from build123d import *

# Parameters (mm, degrees)
SKETCH1_R                                           = 50.375
BOSS_EXTRUDE1_DEPTH                                 = 7
SKETCH3_R                                           = 18.5
CUT_EXTRUDE2_DEPTH                                  = 72.584085173
CBORE_FOR_M3_HEX_SOCKET_HEAD_CAP_SCREW1_D           = 3.4
CBORE_FOR_M3_HEX_SOCKET_HEAD_CAP_SCREW1_CBORE_D     = 6.5
CBORE_FOR_M3_HEX_SOCKET_HEAD_CAP_SCREW1_CBORE_DEPTH = 3.4
CIRPATTERN1_COUNT                                   = 15


with BuildPart() as part:
    # Sketch1 → Boss-Extrude1 (new body)
    with BuildSketch(Plane.XY):
        Circle(SKETCH1_R)
    extrude(amount=BOSS_EXTRUDE1_DEPTH)

    # Sketch3 → Cut-Extrude2 (cut, through all)
    with BuildSketch(Plane.XY.offset(7)):
        Circle(SKETCH3_R)
    extrude(amount=-CUT_EXTRUDE2_DEPTH, mode=Mode.SUBTRACT)

    # CBORE for M3 Hex Socket Head Cap Screw1 (through all)
    with Locations(Plane.XY.offset(7)):
        with Locations((0, 40)):
            cbore_for_m3_hex_socket_head_cap_screw1 = CounterBoreHole(CBORE_FOR_M3_HEX_SOCKET_HEAD_CAP_SCREW1_D / 2, CBORE_FOR_M3_HEX_SOCKET_HEAD_CAP_SCREW1_CBORE_D / 2, CBORE_FOR_M3_HEX_SOCKET_HEAD_CAP_SCREW1_CBORE_DEPTH)

    # CirPattern1: CBORE for M3 Hex Socket Head Cap Screw1 ×15 about axis
    cirpattern1_axis = Axis((0, 0, 0), (0, 0, 1))
    for i in range(1, CIRPATTERN1_COUNT):
        add(cbore_for_m3_hex_socket_head_cap_screw1.rotate(cirpattern1_axis, i * 360 / CIRPATTERN1_COUNT), mode=Mode.SUBTRACT)


solid = part.part
For this review, take the finished solid that the model builds, in its own axes (mm). A direction names the side the tool comes from. Give positions to 0.01 mm unless a question says otherwise; leave off trailing zeros. Order: outer loops, then holes, each group sorted by start corner. A loop starts at its lowest first (then second) coordinate and runs counter-clockwise, first axis right, second up. Notation, with made-up numbers: (-36, 13) - (-19, 13) arc R17 ccw to (-19, 37) - close; hole circle Ø2 at (55.25, 57.25). An arc over 180 degrees is marked (long way). Answer as a JSON object with one key per item and string values. Group by question number.
Item 1: Wall thickness on line 1 along Y through (x, z) = (0, 1.2) (3 decimals); line 2 along X through (y, z) = (9.5, 6.5); line 3 along X through (y, z) = (25.5, 4): over which ranges is each line inside the solid? List them lowest first.
Item 2: Clearance check with flat-ended pins moving along their axes: pin 1 Ø5.5 at (x, y) = (-23.51, -32.36) entering from -Z; pin 2 Ø4 at (x, y) = (0, 40) entering from +Z; pin 3 Ø1.5 at (y, z) = (-33.5, 5.5) entering from -X; pin 4 Ø3 at (x, z) = (-30.5, 2.5) entering from +Y. State where each tip first meets the part, or that it passes through.
Item 3: Take a section at B-B on y = -20. Give the boundary of the cut face in (x, z).
Item 4: Take a section at A-A on x = 0. Give the boundary of the cut face in (y, z) (3 decimals), and give its area (3 significant figures).
Item 5: Machinability: for faces 1 (the cylindrical face through (-13.727, 34.518, 5.324)), 2 (the cylindrical face through (41.434, -4.577, 1.775)), which of the approach directions +Z, -Z, +X, -X, +Y, -Y give a long, thin tool a straight path to every point of the face, cutting with its end or side? Answer none if there is none.
Reported:
{
 "1": {"line 1": "-50.375 to -18.5, 18.5 to 38.3, 41.7 to 50.375", "line 2": "-49.47 to -39.58, -36.5 to -15.87, 15.87 to 36.5, 39.58 to 49.47", "line 3": "-43.44 to -32.72, -26.73 to 26.73, 32.72 to 43.44"},
 "2": {"pin 1": "z = 0", "pin 2": "z = 3.6", "pin 3": "x = -38.28", "pin 4": "y = 41.19"},
 "3": {"outline": "(-46.23, 0) - (-36.34, 0) - (-36.34, 3.6) - (-37.89, 3.6) - (-37.89, 7) - (-46.23, 7) - close; (-32.94, 0) - (32.94, 0) - (32.94, 3.6) - (31.39, 3.6) - (31.39, 7) - (-31.39, 7) - (-31.39, 3.6) - (-32.94, 3.6) - close; (36.34, 0) - (46.23, 0) - (46.23, 7) - (37.89, 7) - (37.89, 3.6) - (36.34, 3.6) - close"},
 "4": {"outline": "(-50.375, 0) - (-18.5, 0) - (-18.5, 7) - (-50.375, 7) - close; (18.5, 0) - (38.3, 0) - (38.3, 3.6) - (36.75, 3.6) - (36.75, 7) - (18.5, 7) - close; (41.7, 0) - (50.375, 0) - (50.375, 7) - (43.25, 7) - (43.25, 3.6) - (41.7, 3.6) - close", "area": "412 mm^2"},
 "5": {"face 1": "+Z", "face 2": "+Z, -Z"}
}
